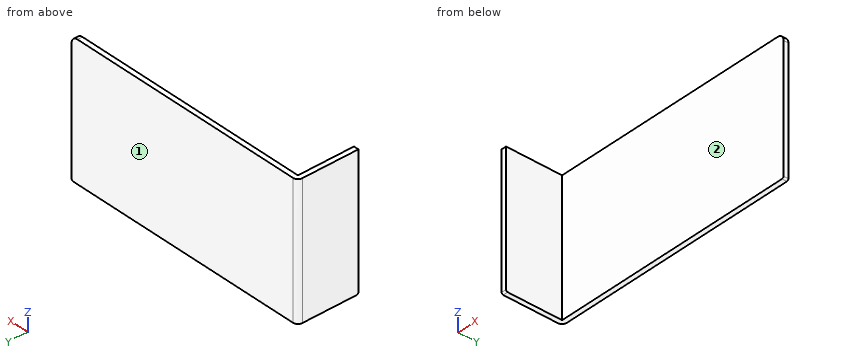
from build123d import *

# Parameters (mm, degrees)
F1_DEPTH = 1.5
F2_W     = 3
F2_H     = 80
F3_DEPTH = 34
F4_R     = 3
F5_R     = 1


with BuildPart() as f1:
    # F0 (on Front) → F1 (new body, symmetric)
    with BuildSketch(Plane.XZ):
        with BuildLine():
            Line((0, 80), (0, 0))
            Line((0, 0), (153, 0))
            Line((153, 0), (153, 76))
            ThreePointArc((153, 76), (151.828427, 78.828427), (149, 80))
            Line((149, 80), (0, 80))
        make_face()
    extrude(amount=F1_DEPTH, both=True)

    # F2 (on face) → F3 (join)
    with BuildSketch(Plane.XZ.offset(1.5)):
        with Locations((1.5, 40)):
            Rectangle(F2_W, F2_H)
    extrude(amount=F3_DEPTH)

    # F4
    f4_edges = [f1.edges().sort_by_distance(p)[0] for p in [
        (0, 1.5, 40),
    ]]
    fillet(f4_edges, radius=F4_R)

    # F5
    f5_edges = [f1.edges().sort_by_distance(p)[0] for p in [
        (1.5, -35.5, 0),
        (153, 0, 0),
    ]]
    fillet(f5_edges, radius=F5_R)


solid = f1.part
Can you work these out from the model? Positions are in its coordinate system, mm. Face numbers are marked on the shaded views. A direction names the side the tool comes from. Give positions to 0.01 mm unless a question says otherwise; leave off trailing zeros. Order: outer loops, then holes, each group sorted by start corner. A loop starts at its lowest first (then second) coordinate and runs counter-clockwise, first axis right, second up. Notation, with made-up numbers: M 64,-36.5 L 78,-36.5 A17 ccw 78,-32.5 Z; hole C 39,17.5 d7. An arc over 180 degrees is marked long. One line per item, written item: value.
Item 1: For pin 1 (2 mm diameter, centred on x = 96.5, z = 65, fed in from -Y); pin 2 (1.5 mm diameter, centred on y = -14, z = 58.5, fed in from +X), each with a flat end and sliding along its axis, tell me the tip position at first contact or that it passes through.
Verdict:
pin 1: y = -1.5
pin 2: x = 3
Item 2: If we section it at A-A on z = 67: Write out the boundary of the cut face in (x, y), and give its area (3 significant figures).
Verdict:
outline: M 0,-35.5 L 3,-35.5 L 3,-1.5 L 153,-1.5 L 153,1.5 L 3,1.5 A3 ccw 0,-1.5 Z
area: 559 mm2
Item 3: If we section it at B-B on x = 11.5: Write out the boundary of the cut face in (y, z), and give its area (3 significant figures).
Verdict:
outline: M -1.5,0 L 1.5,0 L 1.5,80 L -1.5,80 Z
area: 240 mm2
Item 4: Please list where these lines run through material, in increasing order: line 1 (X direction, y = -23, z = 52); line 2 (Y direction, x = 119, z = 15.5).
Verdict:
line 1: 0 to 3
line 2: -1.5 to 1.5
Item 5: For the marked faces 1 and 2, which set-ups out of +Z, -Z, +X, -X, +Y, -Y let a thin tool reach every point of the face, with its end or its side?
Verdict:
face 1: +Z, -Z, +X, -X, +Y
face 2: +Z, -Z, +X, -Y
Item 6: If we section it at C-C on y = -5.5: Write out the boundary of the cut face in (x, z), and give its area (3 significant figures).
Verdict:
outline: M 0,0 L 3,0 L 3,80 L 0,80 Z
area: 240 mm2
